Part model, mm, in its own coordinate system. Round coordinates to 2 decimals unless told otherwise and drop trailing zeros. Write each loop counter-clockwise with the first axis right and the second up, starting at its lowest first coordinate (ties: lowest second). Pieces come first, ordered by that corner, then holes. Notation, with made-up numbers: (-6, -15.5) -> (36, -15.5) arc R30 ccw to (36, 15.5) -> close; hole circle Ø10 at (15.5, 18). An arc over 180 degrees is marked (long way). Return JSON: item names as keys, results as strings. Group by question number.
(1) Drill centre lines: L1, parallel to Y at x = -14, z = 6; L2, parallel to X at y = 194, z = 18.5; L3, parallel to X at y = 233.5, z = 26. Where is each one in solid material? Low to high. Write a range as from..to.
(2) Drop flat-ended pins along their axis: pin 1 Ø1 at (x, z) = (-162.5, 24) entering from -Y; pin 2 Ø4 at (x, y) = (-54, 105.5) entering from +Z; pin 3 Ø1 at (x, z) = (-54, 17.5) entering from +Y. Give the stop position or say it passes through.
(3) Saw through at C-C (z = 8.5). List the corners of the cut face in (x, y), plus the area to 3 significant figures.
(4) Saw through at D-D (z = 42). List the corners of the cut face in (x, y).
(5) Saw through at B-B (x = -46). List the corners of the cut face in (y, z).
(6) Saw through at A-A (y = 50). List the corners of the cut face in (x, z), plus the area to 3 significant figures.
from build123d import *

# Parameters (mm, degrees)
F0_R     = 7
F1_DEPTH = 25
F2_DEPTH = 50


with BuildPart() as f1:
    # F0 (on Top) → F1 (new body)
    with BuildSketch(Plane.XY):
        with BuildLine():
            Line((-151.999996, -0.034339), (0, 0))
            Line((0, 0), (0, 200))
            ThreePointArc((0, 200), (-38.319968, 151.383369), (-94.543074, 177.286247))
            ThreePointArc((-94.543074, 177.286247), (-93.668792, 133.66164), (-127.382019, 105.961658))
            Line((-127.382019, 105.961658), (-303.277156, 63.611034))
            ThreePointArc((-303.277156, 63.611034), (-291.336288, 60.997277), (-286, 50))
            ThreePointArc((-286, 50), (-291.336288, 39.002723), (-303.277156, 36.388966))
            Line((-303.277156, 36.388966), (-151.999996, -0.034339))
        make_face()
        with Locations((-14, 14)):
            Circle(F0_R, mode=Mode.SUBTRACT)
        with BuildLine():
            ThreePointArc((-303.277156, 63.611034), (-314, 50), (-303.277156, 36.388966))
            ThreePointArc((-303.277156, 36.388966), (-291.336288, 39.002723), (-286, 50))
            ThreePointArc((-286, 50), (-291.336288, 60.997277), (-303.277156, 63.611034))
        make_face()
        with Locations((-300, 50)):
            Circle(F0_R, mode=Mode.SUBTRACT)
    extrude(amount=F1_DEPTH)

    # F0 (on Top) → F2 (join)
    with BuildSketch(Plane.XY):
        with BuildLine():
            ThreePointArc((-94.543074, 177.286247), (-38.319968, 151.383369), (0, 200))
            ThreePointArc((0, 200), (-14.644661, 235.355339), (-50, 250))
            ThreePointArc((-50, 250), (-92.63618, 226.11812), (-94.543074, 177.286247))
        make_face()
        with BuildLine():
            ThreePointArc((-84.641016, 180), (-86.955181, 184.692663), (-88.637033, 189.647238))
            ThreePointArc((-88.637033, 189.647238), (-85.101499, 195.770963), (-78.977775, 192.235429))
            ThreePointArc((-78.977775, 192.235429), (-75.980762, 185), (-71.213203, 178.786797))
            ThreePointArc((-71.213203, 178.786797), (-71.213203, 171.715729), (-78.284271, 171.715729))
            ThreePointArc((-78.284271, 171.715729), (-81.734134, 175.649543), (-84.641016, 180))
        make_face(mode=Mode.SUBTRACT)
        with BuildLine():
            ThreePointArc((-15.358984, 180), (-18.265866, 175.649543), (-21.715729, 171.715729))
            ThreePointArc((-21.715729, 171.715729), (-28.786797, 171.715729), (-28.786797, 178.786797))
            ThreePointArc((-28.786797, 178.786797), (-24.019238, 185), (-21.022225, 192.235429))
            ThreePointArc((-21.022225, 192.235429), (-14.898501, 195.770963), (-11.362967, 189.647238))
            ThreePointArc((-11.362967, 189.647238), (-13.044819, 184.692663), (-15.358984, 180))
        make_face(mode=Mode.SUBTRACT)
        with BuildLine():
            ThreePointArc((-60.352762, 238.637033), (-55.221048, 239.657794), (-50, 240))
            ThreePointArc((-50, 240), (-44.778952, 239.657794), (-39.647238, 238.637033))
            ThreePointArc((-39.647238, 238.637033), (-36.111704, 232.513309), (-42.235429, 228.977775))
            ThreePointArc((-42.235429, 228.977775), (-46.084214, 229.743346), (-50, 230))
            ThreePointArc((-50, 230), (-53.915786, 229.743346), (-57.764571, 228.977775))
            ThreePointArc((-57.764571, 228.977775), (-63.888296, 232.513309), (-60.352762, 238.637033))
        make_face(mode=Mode.SUBTRACT)
    extrude(amount=F2_DEPTH)


solid = f1.part
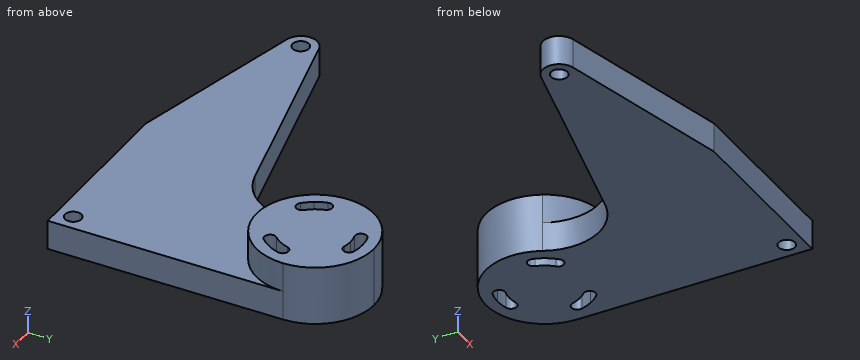
Computed values:
{
 "1": {"L1": "0..7, 21..182.56, 195.43..234.7", "L2": "-99.64..-87.76, -79.85..-20.15, -12.24..0", "L3": "-87.12..-64.05, -35.95..-12.88"},
 "2": {"pin 1": "y = 2.37", "pin 2": "z = 25", "pin 3": "y = 249.88"},
 "3": {"outline": "(-303.28, 36.39) -> (-152, -0.03) -> (0, 0) -> (0, 200) arc R50 ccw (long way) to (-94.54, 177.29) arc R50 cw to (-127.38, 105.96) -> (-303.28, 63.61) arc R14 ccw to start; hole circle Ø14 at (-300, 50); hole (-88.64, 189.65) arc R40 ccw to (-84.64, 180) arc R40 ccw to (-78.28, 171.72) arc R5 ccw to (-71.21, 178.79) arc R30 cw to (-78.98, 192.24) arc R5 ccw to start; hole (-60.35, 238.64) arc R5 ccw to (-57.76, 228.98) arc R30 cw to (-50, 230) arc R30 cw to (-42.24, 228.98) arc R5 ccw to (-39.65, 238.64) arc R40 ccw to (-50, 240) arc R40 ccw to start; hole (-28.79, 178.79) arc R5 ccw to (-21.72, 171.72) arc R40 ccw to (-15.36, 180) arc R40 ccw to (-11.36, 189.65) arc R5 ccw to (-21.02, 192.24) arc R30 cw to start; hole circle Ø14 at (-14, 14)", "area": "37,800 mm2"},
 "4": {"outline": "circle Ø100 at (-50, 200); hole (-88.64, 189.65) arc R40 ccw to (-84.64, 180) arc R40 ccw to (-78.28, 171.72) arc R5 ccw to (-71.21, 178.79) arc R30 cw to (-78.98, 192.24) arc R5 ccw to start; hole (-60.35, 238.64) arc R5 ccw to (-57.76, 228.98) arc R30 cw to (-50, 230) arc R30 cw to (-42.24, 228.98) arc R5 ccw to (-39.65, 238.64) arc R40 ccw to (-50, 240) arc R40 ccw to start; hole (-28.79, 178.79) arc R5 ccw to (-21.72, 171.72) arc R40 ccw to (-15.36, 180) arc R40 ccw to (-11.36, 189.65) arc R5 ccw to (-21.02, 192.24) arc R30 cw to start"},
 "5": {"outline": "(-0.01, 0) -> (229.73, 0) -> (229.73, 50) -> (150.16, 50) -> (150.16, 25) -> (-0.01, 25) -> close; (239.8, 0) -> (249.84, 0) -> (249.84, 50) -> (239.8, 50) -> close"},
 "6": {"outline": "(-314, 0) -> (-307, 0) -> (-307, 25) -> (-314, 25) -> close; (-293, 0) -> (0, 0) -> (0, 25) -> (-293, 25) -> close", "area": "7,500 mm2"}
}
